Source: three-view drawing plus pictorial views. Frame: mm from the lowest corner of the part. A direction names the side the tool comes from. Round coordinates to 2 decimals unless told otherwise and drop trailing zeros. Order: outer loops, then holes, each group sorted by start corner. A loop starts at its lowest first (then second) coordinate and runs counter-clockwise, first axis right, second up. Notation, with made-up numbers: (77.25, -8) -> (85.25, -8) arc R26 cw to (85.25, 31) -> close; hole circle Ø2 at (25, 2.5). An arc over 180 degrees is marked (long way). Use a Markdown table: item, result.
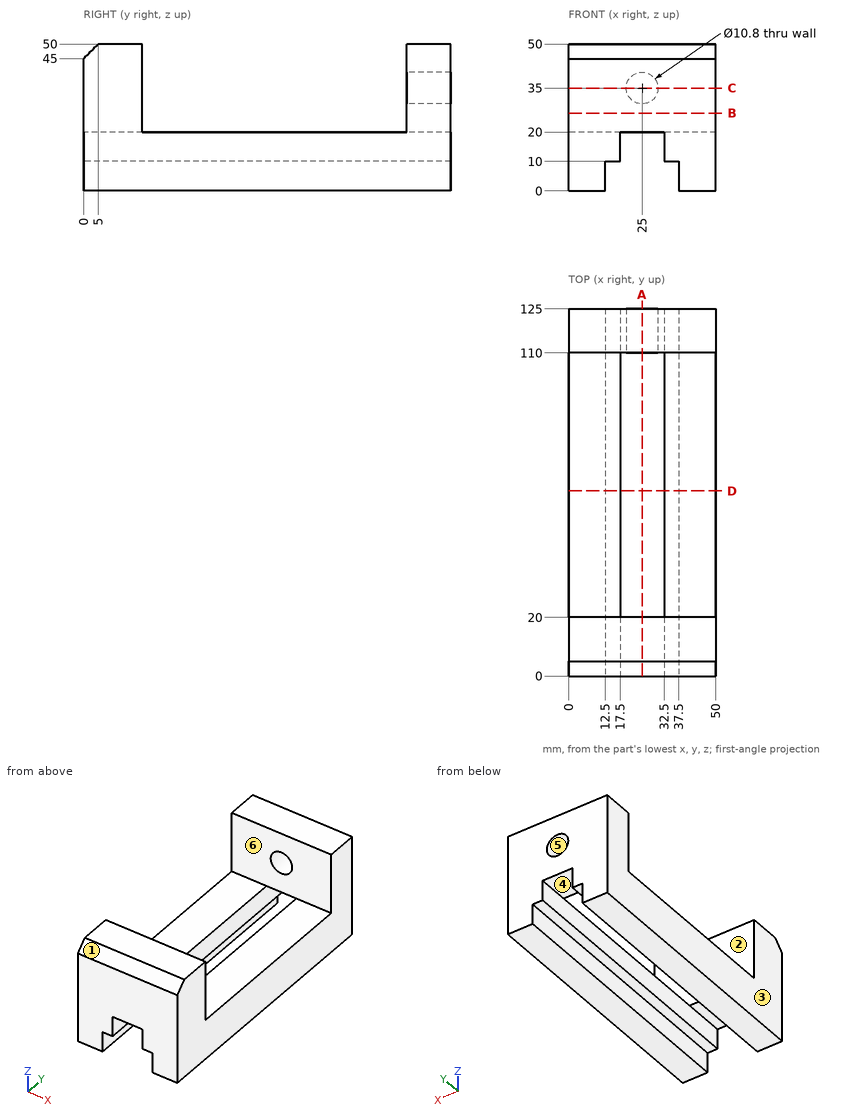
1) Pin query (flat end, axial travel): pin 1 Ø7.5 at (x, y) = (23, 12) entering from -Z; pin 2 Ø10 at (x, y) = (28.5, 105) entering from -Z; pin 3 Ø9 at (x, y) = (7.5, 67.5) entering from +Z; pin 4 Ø12 at (x, y) = (25.5, 26.5) entering from +Z. Return the tip coordinate at first contact, or that it passes through.
Results found:
| item | result |
|---|---|
| pin 1 | stops at z = 20 |
| pin 2 | stops at z = 10 |
| pin 3 | stops at z = 20 |
| pin 4 | passes through |
2) Cut plane B-B on z = 26.5. Return loops of the section in (x, y), and give its area (3 significant figures).
Results found:
| item | result |
|---|---|
| outline | (0, 0) -> (50, 0) -> (50, 20) -> (0, 20) -> close; (0, 110) -> (50, 110) -> (50, 125) -> (0, 125) -> close |
| area | 1,750 mm² |
3) Set-up query: the marked faces 4, 5 and 6. Return all of +Z, -Z, +X, -X, +Y, -Y with unobstructed straight access to the full face (end or side cutting, diameter ignored); none if empty.
Results found:
| item | result |
|---|---|
| face 4 | -Z, +Y, -Y |
| face 5 | +Y |
| face 6 | +Z, +X, -X |
4) Line query: L1, parallel to Y at x = 44, z = 23; L2, parallel to Z at x = 25, y = 119.5; L3, parallel to X at y = 117.25, z = 35. Output: solid intervals per line, ascending. Write a range as [from, to].
Results found:
| item | result |
|---|---|
| L1 | y = [0, 20], [110, 125] |
| L2 | z = [20, 29.6], [40.4, 50] |
| L3 | x = [0, 19.6], [30.4, 50] |
5) Pull-direction query (Y, two-part tool) for the marked faces 1, 2 and 3; classes: +Y half, -Y half, draft (parallel to the pull), parting line (faces both ways), or undercut.
Results found:
| item | result |
|---|---|
| face 1 | -Y half |
| face 2 | undercut |
| face 3 | draft |
6) Cut plane C-C on z = 35. Return loops of the section in (x, y).
Results found:
| item | result |
|---|---|
| outline | (0, 0) -> (50, 0) -> (50, 20) -> (0, 20) -> close; (0, 110) -> (19.6, 110) -> (19.6, 125) -> (0, 125) -> close; (30.4, 110) -> (50, 110) -> (50, 125) -> (30.4, 125) -> close |
7) Cut plane A-A on x = 25. Return loops of the section in (y, z).
Results found:
| item | result |
|---|---|
| outline | (0, 20) -> (20, 20) -> (20, 50) -> (5, 50) -> (0, 45) -> close; (110, 20) -> (125, 20) -> (125, 29.6) -> (110, 29.6) -> close; (110, 40.4) -> (125, 40.4) -> (125, 50) -> (110, 50) -> close |
8) Cut plane D-D on y = 63. Return loops of the section in (x, z), and give its area (3 significant figures).
Results found:
| item | result |
|---|---|
| outline | (0, 0) -> (12.5, 0) -> (12.5, 10) -> (17.5, 10) -> (17.5, 20) -> (0, 20) -> close; (32.5, 10) -> (37.5, 10) -> (37.5, 0) -> (50, 0) -> (50, 20) -> (32.5, 20) -> close |
| area | 600 mm² |
